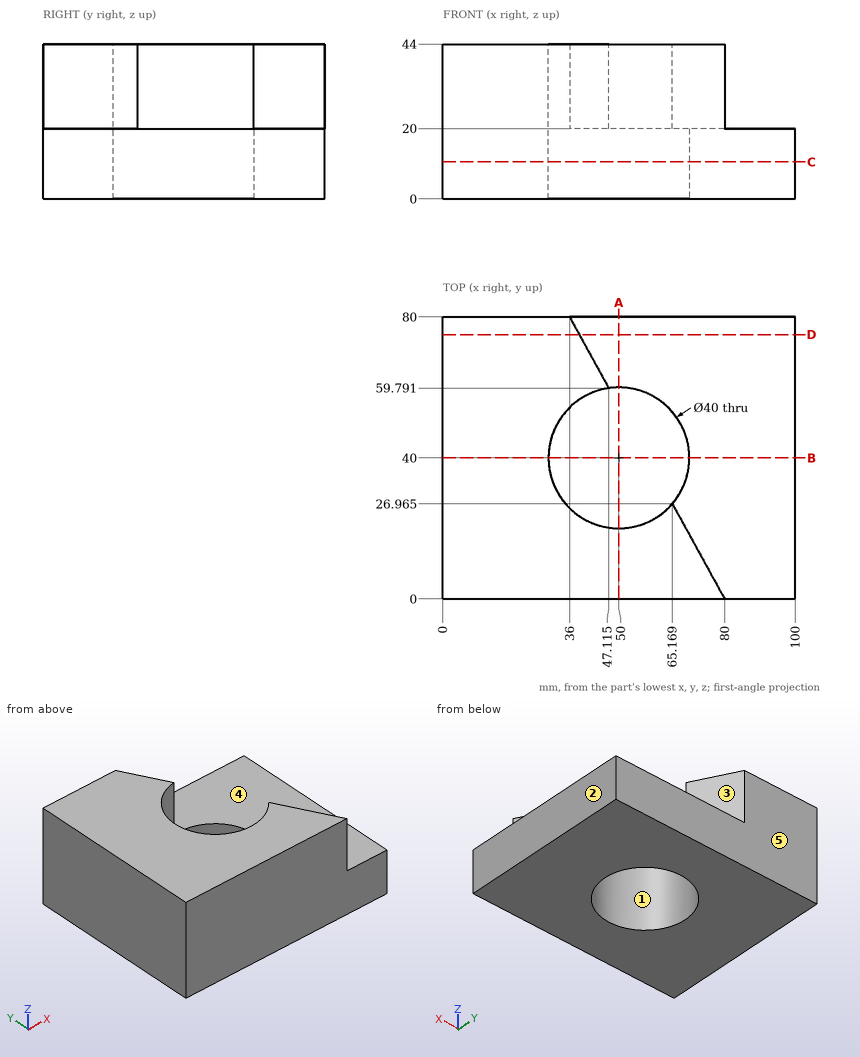
Check sheet for the drawn part. Datum: minimum x, y, z corner. Units: mm. A direction names the side the tool comes from. Give positions to 0.01 mm unless a question says otherwise; leave off trailing zeros. Loops run counter-clockwise (first coordinate to the right, second up) from the corner with the lowest first, then second, coordinate; pieces in that order, holes last.
1) Draft check along Y on the marked faces 1, 2 and 3. Enter one of: pulls with the +Y half, pulls with the -Y half, needs draft (parallel to the pull), parting line crosses it, or undercut.
2) Sectioned sample at D-D, the plane y = 75. Enter the section's corners in (x, z).
3) Set-up check for the marked faces 4 and 5: record each of +Z, -Z, +X, -X, +Y, -Y from which the full face is reachable in a straight line by a thin tool's end or side.
4) Sectioned sample at A-A, the plane x = 50. Enter the section's corners in (y, z).
5) Sectioned sample at B-B, the plane y = 40. Enter the section's corners in (x, z).
6) Thickness scan on line 1 along Y through (x, z) = (49.5, 3.5); line 2 along X through (y, z) = (40, 9); line 3 along Z through (x, y) = (83, 27). Record the ranges inside material, lowest first.
7) Sectioned sample at C-C, the plane z = 10.5. Enter the section's corners in (x, y).
8) Depth check by flat-ended pin: pin 1 Ø6 at (y, z) = (71, 37) entering from +X; pin 2 Ø6 at (x, y) = (86.5, 40.5) entering from +Z; pin 3 Ø1 at (y, z) = (56, 31.5) entering from +X. Enter the tip coordinate at first touch or a pass-through.
Answers:
1. face 1: undercut
1. face 2: needs draft
1. face 3: pulls with the +Y half
2. outline: (0, 0) - (100, 0) - (100, 20) - (38.75, 20) - (38.75, 44) - (0, 44) - close
3. face 4: +Z, +X, +Y
3. face 5: +Z, -Z, +X, -X, +Y
4. outline: (0, 0) - (20, 0) - (20, 44) - (0, 44) - close; (60, 0) - (80, 0) - (80, 20) - (60, 20) - close
5. outline: (0, 0) - (30, 0) - (30, 44) - (0, 44) - close; (70, 0) - (100, 0) - (100, 20) - (70, 20) - close
6. line 1: y = 0 to 20.01, 59.99 to 80
6. line 2: x = 0 to 30, 70 to 100
6. line 3: z = 0 to 20
7. outline: (0, 0) - (100, 0) - (100, 80) - (0, 80) - close; hole circle Ø40 at (50, 40)
8. pin 1: stops at x = 42.6
8. pin 2: stops at z = 20
8. pin 3: stops at x = 38.7
